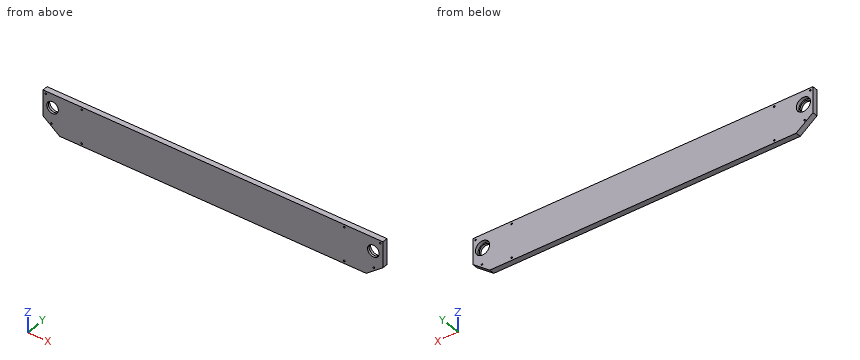
```python
from build123d import *

# Parameters (mm, degrees)
F0_R     = 3
F0_R_2   = 27.5
F1_DEPTH = 21
F2_R     = 27.5
F2_R_2   = 22.5
F3_DEPTH = 8


# Not quite as in the source:
# - a feature names something its author has since deleted; it is built from what else it names


with BuildPart() as f1:
    # F0 (on Front) → F1 (new body)
    with BuildSketch(Plane.XZ):
        Polygon((0, 50), (65, 0), (160, 0), (1255.0009576903, 0), (1320, 50), (1320, 150), (160, 150), (0, 150), (0, 120), align=None)
        with Locations((150, 10)):
            Circle(F0_R, mode=Mode.SUBTRACT)
        with Locations((32.5, 35)):
            Circle(F0_R, mode=Mode.SUBTRACT)
        with Locations((1170, 10)):
            Circle(F0_R, mode=Mode.SUBTRACT)
        with Locations((1285, 35)):
            Circle(F0_R, mode=Mode.SUBTRACT)
        with Locations((37, 98)):
            Circle(F0_R_2, mode=Mode.SUBTRACT)
        with Locations((10, 140)):
            Circle(F0_R, mode=Mode.SUBTRACT)
        with Locations((150, 140)):
            Circle(F0_R, mode=Mode.SUBTRACT)
        with Locations((1283, 98)):
            Circle(F0_R_2, mode=Mode.SUBTRACT)
        with Locations((1170, 140)):
            Circle(F0_R, mode=Mode.SUBTRACT)
        with Locations((1310, 140)):
            Circle(F0_R, mode=Mode.SUBTRACT)
    extrude(amount=-F1_DEPTH)

    # F2 (on face) → F3 (join)
    with BuildSketch(Plane.XZ):
        with Locations((1283, 98)):
            Circle(F2_R)
        with Locations((1283, 98)):
            Circle(F2_R_2, mode=Mode.SUBTRACT)
        with Locations((37, 98)):
            Circle(F2_R)
        with Locations((37, 98)):
            Circle(F2_R_2, mode=Mode.SUBTRACT)
    extrude(amount=-F3_DEPTH)


solid = f1.part
```
Check sheet for the modelled part. Datum: model origin and axes. Units: mm. Round coordinates to 2 decimals unless told otherwise and drop trailing zeros. One line per item, written item: value. Start each with the question number.
Q1. Cross-section at A-A (y = 17.75). Give the number of separate pieces and of enclosed holes in the cut face, and give its area (3 significant figures).
Q2. Gauge pin test, flat ends, axial feed: pin 1 Ø5.5 at (x, z) = (150, 10) entering from +Y; pin 2 Ø5 at (y, z) = (3, 17) entering from +X. Record the tip position at first contact, or that the pin passes through.
Q3. Thickness scan on line 1 (X direction, y = 13.75, z = 140); line 2 (Z direction, x = 150, y = 10.25); line 3 (Z direction, x = 32.5, y = 7.5). Record the ranges inside material, lowest first.
Completed:
1. separate pieces: 1
1. enclosed holes: 10
1. area: 190,000 mm²
2. pin 1: passes through
2. pin 2: stops at x = 1280.35
3. line 1: x = 0 to 7, 13 to 147, 153 to 1167, 1173 to 1307, 1313 to 1320
3. line 2: z = 0 to 7, 13 to 137, 143 to 150
3. line 3: z = 25 to 32, 38 to 75.95, 120.05 to 150
